from build123d import *

# Parameters (mm, degrees)
F1_DEPTH        = 3
F2_W            = 26.8
F2_H            = 30
F3_DEPTH        = 5
F4_W            = 26.8
F4_H            = 30
F5_DEPTH        = 14
F7_DEPTH        = 12.7
F8_W            = 6.35
F8_H            = 1
F9_DEPTH        = 10
F10_R           = 2.5
F11_SIZE        = 1.27
F13_D           = 2.2606
F13_DEPTH       = 14.61135
F13_CSINK_D     = 6.477
F13_CSINK_ANGLE = 82
F13_TIP         = 0.6791527577


with BuildPart() as f1:
    # F0 (on Front) → F1 (new body)
    with BuildSketch(Plane.XZ):
        Polygon((13.5, 16.5), (-13.5, 16.5), (-22, 0), (-13.5, -16.5), (13.5, -16.5), (22, 0), align=None)
    extrude(amount=F1_DEPTH)

    # F2 (on face) → F3 (join)
    with BuildSketch(Plane(origin=(0, 0, 0), x_dir=(-1, 0, 0), z_dir=(0, 1, 0))):
        Rectangle(F2_W, F2_H)
    extrude(amount=-F3_DEPTH)

    # F4 (on face) → F5 (join)
    with BuildSketch(Plane(origin=(0, 0, 0), x_dir=(-1, 0, 0), z_dir=(0, 1, 0))):
        Rectangle(F4_W, F4_H)
    extrude(amount=F5_DEPTH)

    # F6 (on face) → F7 (cut)
    with BuildSketch(Plane.XZ.offset(5)):
        Polygon((-12, 8.3), (-12, -2.7), (12, -2.7), (12, 8.3), (7, 13.3), (-7, 13.3), align=None)
    extrude(amount=-F7_DEPTH, mode=Mode.SUBTRACT)

    # F8 (on face) → F9 (join)
    with BuildSketch(Plane(origin=(0, 14, 0), x_dir=(-1, 0, 0), z_dir=(0, 1, 0))):
        with Locations((0, 10.3100380624)):
            Rectangle(F8_W, F8_H)
        with Locations((-7.7292244386, 0)):
            Rectangle(F8_W, F8_H)
        with Locations((-7.5456485327, -10.9369392929)):
            Rectangle(F8_W, F8_H)
    extrude(amount=F9_DEPTH)

    # F10
    f10_edges = [f1.edges().sort_by_distance(p)[0] for p in [
        (-22, -1.5, 0),
        (-13.5, -1.5, 16.5),
        (13.5, -1.5, 16.5),
        (22, -1.5, 0),
        (13.5, -1.5, -16.5),
        (-13.5, -1.5, -16.5),
        (-13.4, -4, -15),
        (13.4, -4, -15),
        (13.4, -4, 15),
        (-13.4, -4, 15),
        (-13.4, 7, 15),
        (13.4, 7, 15),
        (-13.4, 7, -15),
        (13.4, 7, -15),
        (-12, 1.35, 8.3),
        (-7, 1.35, 13.3),
        (7, 1.35, 13.3),
        (12, 1.35, 8.3),
        (12, 1.35, -2.7),
        (-12, 1.35, -2.7),
    ]]
    fillet(f10_edges, radius=F10_R)

    # F11
    f11_edges = [f1.edges().sort_by_distance(p)[0] for p in [
        (10.720649, 24, -10.936939),
        (10.904224, 24, 0),
        (3.175, 24, 10.310038),
        (-3.175, 24, 10.310038),
        (4.554224, 24, 0),
        (4.370649, 24, -10.936939),
    ]]
    chamfer(f11_edges, length=F11_SIZE)

    # F13
    with Locations(Plane.XZ.offset(3)):
        with Locations((-18, 0), (18, 0)):
            CounterSinkHole(F13_D / 2, F13_CSINK_D / 2, depth=F13_DEPTH, counter_sink_angle=F13_CSINK_ANGLE)
            with Locations((0, 0, -(F13_DEPTH + F13_TIP / 2))):  # 118° drill point
                Cone(0, F13_D / 2, F13_TIP, mode=Mode.SUBTRACT)


solid = f1.part
Can you work these out from the model? Positions are in its coordinate system, mm. A direction names the side the tool comes from. Coordinates: 2 decimals unless noted, no trailing zeros. Order: outer loops, then holes, each group sorted by start corner. A loop starts at its lowest first (then second) coordinate and runs counter-clockwise, first axis right, second up. Notation, with made-up numbers: (75.25, 74.5) - (128.25, 74.5) arc R21 ccw to (128.25, 102.5) - close; hole circle Ø2 at (52.25, 81). An arc over 180 degrees is marked (long way). Answer as a JSON object with one key per item and string values. Group by question number.
Q1. Imagine slicing it at D-D (y = 8.75). Please give me the cut outline in (x, z).
Q2. On a 3-axis mill with a long thin cutter (end or side, diameter ignored), from which of +Z, -Z, +X, -X, +Y, -Y can I reach the whole of each face in a straight line? I mean faces 5 (the face through (10.08, 23.37, -10.94)), 6 (the face through (0, 19, 9.81)), 7 (the face through (11.804, 1.439, 8.234)), 8 (the face through (12.648, -4.014, 14.287)). Say none if no direction works.
Q3. Imagine slicing it at C-C (z = -4.5). Please give me the cut outline in (x, y), and give its area (3 significant figures).
Q4. Imagine slicing it at A-A (y = 2). Please give me the cut outline in (x, z), and give its area (3 significant figures).
Q5. Will these pins go through, and if not, where does the flat tip stop? P1, Ø0.5, axis at y = 18.5, z = 10.5, coming from the -X side (3 decimals); P2, Ø10, axis at x = -5.5, z = 2.5, coming from the +Y side; P3, Ø6, axis at x = 16, y = 8.5, coming from the -Z side; P4, Ø2, axis at x = 18, z = 0, coming from the -Y side.
Q6. Imagine slicing it at B-B (x = -18). Please give me the cut outline in (y, z).
Q7. I need wall thicknesses on line 1 (X direction, y = -0.4, z = 0); line 2 (X direction, y = 7.25, z = 3); line 3 (Y direction, x = 18, z = 6.5). Which ranges of each line are inside material? Lowest first, please. Write a range as from..to.
Q8. We'd pull the mould along X, two halves only. Please class faces 1 (the face through (-11.804, 1.439, 8.234)), 2 (the face through (-17.855, -1.479, -8.047)), 3 (the face through (14, -3, 0)), 4 (the face through (0, 1, -2.7)): +X half, -X half, draft (parallel to the pull), parting line (faces both ways), or undercut.
Determined:
{
 "1": {"outline": "(-13.4, -12.5) arc R2.5 ccw to (-10.9, -15) - (10.9, -15) arc R2.5 ccw to (13.4, -12.5) - (13.4, 12.5) arc R2.5 ccw to (10.9, 15) - (-10.9, 15) arc R2.5 ccw to (-13.4, 12.5) - close"},
 "2": {"face 5": "-Z, +X, +Y", "face 6": "-Z, +X, -X, +Y", "face 7": "-Y", "face 8": "+Z, +X, -Y"},
 "3": {"outline": "(-19.68, -3) - (-13.4, -3) - (-13.4, -5) - (13.4, -5) - (13.4, -3) - (19.68, -3) - (19.68, 0) - (13.4, 0) - (13.4, 14) - (-13.4, 14) - (-13.4, 0) - (-19.68, 0) - close", "area": "547 mm2"},
 "4": {"outline": "(-13.4, -12.5) arc R2.5 ccw to (-10.9, -15) - (10.9, -15) arc R2.5 ccw to (13.4, -12.5) - (13.4, 12.5) arc R2.5 ccw to (10.9, 15) - (-10.9, 15) arc R2.5 ccw to (-13.4, 12.5) - close; hole (-12, -0.2) arc R2.5 ccw to (-9.5, -2.7) - (9.5, -2.7) arc R2.5 ccw to (12, -0.2) - (12, 7.26) arc R2.5 ccw to (11.27, 9.03) - (7.73, 12.57) arc R2.5 ccw to (5.96, 13.3) - (-5.96, 13.3) arc R2.5 ccw to (-7.73, 12.57) - (-11.27, 9.03) arc R2.5 ccw to (-12, 7.26) - close", "area": "443 mm2"},
 "5": {"P1": "stops at x = -3.175", "P2": "stops at y = 14", "P3": "stops at z = -13.86", "P4": "passes through"},
 "6": {"outline": "(-3, -7.76) - (0, -7.76) - (0, -1.13) - (-0.57, -1.13) - (-3, -3.24) - close; (-3, 3.24) - (-0.57, 1.13) - (0, 1.13) - (0, 7.76) - (-3, 7.76) - close"},
 "7": {"line 1": "x = -21.69..-19.13, -16.87..-12, 12..16.87, 19.13..21.69", "line 2": "x = -13.4..-12, 12..13.4", "line 3": "y = -3..0"},
 "8": {"face 1": "undercut", "face 2": "-X half", "face 3": "draft", "face 4": "undercut"}
}
